Build history of the part. All positions in model axes, mm. A direction names the side the tool comes from. Round coordinates to 2 decimals unless told otherwise and drop trailing zeros. Write each loop counter-clockwise with the first axis right and the second up, starting at its lowest first coordinate (ties: lowest second). Pieces come first, ordered by that corner, then holes.
from build123d import *

# Parameters (mm, degrees)
SKETCH1_W           = 16
SKETCH1_H           = 16
SKETCH1_W_2         = 12
SKETCH1_H_2         = 12
BOSS_EXTRUDE1_DEPTH = 240
FILLET1_R           = 1
SKETCH2_R           = 1.75
CUT_EXTRUDE1_DEPTH  = 20
SKETCH3_R           = 2
CUT_EXTRUDE2_DEPTH  = 20


with BuildPart() as part:
    # Sketch1 → Boss-Extrude1 (new body)
    with BuildSketch(Plane(origin=(0, 0, 0), x_dir=(1, 0, 0), z_dir=(0, 1, 0))):
        with Locations((2.245614035, -1.684210526)):
            Rectangle(SKETCH1_W, SKETCH1_H)
        with Locations((2.245614035, -1.684210526)):
            Rectangle(SKETCH1_W_2, SKETCH1_H_2, mode=Mode.SUBTRACT)
    extrude(amount=BOSS_EXTRUDE1_DEPTH)

    # Fillet1
    fillet1_edges = [part.edges().sort_by_distance(p)[0] for p in [
        (-5.754385965, 120, -6.315789474),
        (10.245614035, 120, -6.315789474),
        (10.245614035, 120, 9.684210526),
        (-5.754385965, 120, 9.684210526),
    ]]
    fillet(fillet1_edges, radius=FILLET1_R)

    # Sketch2 → Cut-Extrude1 (cut)
    with BuildSketch(Plane(origin=(10.245614035, 0, 0), x_dir=(0, 0, -1), z_dir=(1, 0, 0))):
        with Locations((-1.684210526, 35.25)):
            Circle(SKETCH2_R)
        with Locations((-1.684210526, 5.25)):
            Circle(SKETCH2_R)
        with Locations((-1.684210526, 20.25)):
            Circle(SKETCH2_R)
    extrude(amount=-CUT_EXTRUDE1_DEPTH, mode=Mode.SUBTRACT)

    # Sketch3 → Cut-Extrude2 (cut)
    with BuildSketch(Plane(origin=(10.245614035, 0, 0), x_dir=(0, 0, -1), z_dir=(1, 0, 0))):
        with Locations((-1.684210526, 60)):
            Circle(SKETCH3_R)
        with Locations((-1.684210526, 50)):
            Circle(SKETCH3_R)
    extrude(amount=-CUT_EXTRUDE2_DEPTH, mode=Mode.SUBTRACT)


solid = part.part
1) Slice it at A-A (x = -1.5). Write the cut outline in (y, z).
Results:
outline: (0, -6.32) - (240, -6.32) - (240, -4.32) - (0, -4.32) - close; (0, 7.68) - (240, 7.68) - (240, 9.68) - (0, 9.68) - close
2) Slice it at C-C (y = 50). Write the cut outline in (x, z).
Results:
outline: (-5.75, -5.32) arc R1 ccw to (-4.75, -6.32) - (9.25, -6.32) arc R1 ccw to (10.25, -5.32) - (10.25, -0.32) - (8.25, -0.32) - (8.25, -4.32) - (-3.75, -4.32) - (-3.75, -0.32) - (-5.75, -0.32) - close; (-5.75, 3.68) - (-3.75, 3.68) - (-3.75, 7.68) - (8.25, 7.68) - (8.25, 3.68) - (10.25, 3.68) - (10.25, 8.68) arc R1 ccw to (9.25, 9.68) - (-4.75, 9.68) arc R1 ccw to (-5.75, 8.68) - close
3) Slice it at D-D (y = 136). Write the cut outline in (x, z), plus the area to 3 significant figures.
Results:
outline: (-5.75, -5.32) arc R1 ccw to (-4.75, -6.32) - (9.25, -6.32) arc R1 ccw to (10.25, -5.32) - (10.25, 8.68) arc R1 ccw to (9.25, 9.68) - (-4.75, 9.68) arc R1 ccw to (-5.75, 8.68) - close; hole (-3.75, -4.32) - (8.25, -4.32) - (8.25, 7.68) - (-3.75, 7.68) - close
area: 111 mm2
4) Slice it at B-B (z = -2.25). Write the cut outline in (x, y), plus the area to 3 significant figures.
Results:
outline: (-5.75, 0) - (-3.75, 0) - (-3.75, 240) - (-5.75, 240) - close; (8.25, 0) - (10.25, 0) - (10.25, 240) - (8.25, 240) - close
area: 960 mm2
5) Mould opens along Z. For faces 1 (the cylindrical face through (9.26, 61.983, 1.945)), 2 (the flat face through (2, 118, 9.684)), 3 (the flat face through (-5, 0, 2)) say: released by +Z, released by -Z, zero draft, split by the parting line, or undercut.
Results:
face 1: undercut
face 2: released by +Z
face 3: zero draft
6) Which spindle directions (+Z, -Z, +X, -X, +Y, -Y) get a long thin tool onto all of the face, cutting with end or side? Do faces 4 (the flat face through (8.246, 118, 2)), 5 (the flat face through (10.246, 118, 2)). Say none if no direction does.
Results:
face 4: +Y, -Y
face 5: +Z, -Z, +X, +Y, -Y
7) Wall check: L1, parallel to X at y = 79, z = -2.75; L2, parallel to Z at x = 0.5, y = 188.5. Give the ranges that are in metal, low to high.
Results:
L1: x = -5.75 to -3.75, 8.25 to 10.25
L2: z = -6.32 to -4.32, 7.68 to 9.68
